Autodesk Inventor part; units mm, degrees
ref_plane "YZ Plane" through (0, 0, 0) normal (1, 0, 0) x (0, 1, 0)
ref_plane "XZ Plane" through (0, 0, 0) normal (0, 1, 0) x (-1, 0, 0)
ref_plane "XY Plane" through (0, 0, 0) normal (0, 0, 1) x (1, 0, 0)
sketch "スケッチ1" plane through (0, 0, 0) normal (0, 0, 1) x (1, 0, 0)
  circle A0 centre (-11.4931, -19.1593) radius 14 construction
  circle A1 centre (16.245, -15.3385) radius 14 construction
  line L0 (-170.915, -81.4118) -> (490.0044, -81.4118)
  line L1 (-197.2268, -33.1593) -> (179.6604, -33.1593) construction
  line L2 (-178.6504, 68.5882) -> (447.0756, 68.5882) construction
  circle A2 centre (-11.4931, -19.1593) radius 14 construction
  circle A3 centre (-21.8854, 6.8407) radius 14 construction
  circle A4 centre (-0.5211, 0.3031) radius 20.05 construction
  circle A5 centre (-0.5211, 0.3031) radius 22.3421 construction
  circle A6 centre (0, 0) radius 22.3421 construction
  circle A7 centre (-0.5211, 0.3031) radius 5.05 construction
  circle A8 centre (19.689, 29.6103) radius 30.55 construction
  circle A9 centre (19.689, 29.6103) radius 10.1 construction
  circle A10 centre (39.672, 58.5882) radius 25.1 construction
  line L3 (-0.5211, 0.3031) -> (39.672, 58.5882) construction
  circle A11 centre (19.689, 29.6103) radius 31.55 construction
  circle A12 centre (19.689, 29.6103) radius 12.1 construction
  circle A13 centre (-0.5211, 0.3031) radius 20.55 construction
  circle A14 centre (-0.5211, 0.3031) radius 6.05 construction
  circle A15 centre (36.8436, 61.4166) radius 4 construction
  circle A16 centre (36.8436, 61.4166) radius 2
  line L4 (36.8436, 61.4166) -> (39.672, 58.5882)
  line L5 (39.672, 58.5882) -> (22.909, 61.4166) construction
  circle A17 centre (22.909, 61.4166) radius 2
  circle A18 centre (22.909, 61.4166) radius 5
  line L6 (28.2635, 50.4737) -> (31.5576, 69.9968) construction
  line L7 (31.5576, 69.9968) -> (51.0806, 66.7027) construction
  line L8 (51.0806, 66.7027) -> (47.7865, 47.1796) construction
  line L9 (47.7865, 47.1796) -> (28.2635, 50.4737) construction
  circle A19 centre (39.672, 58.5882) radius 9
  circle A20 centre (28.2635, 50.4737) radius 2.5
  circle A21 centre (47.7865, 47.1796) radius 2.5
  circle A22 centre (51.0806, 66.7027) radius 2.5
  circle A23 centre (31.5576, 69.9968) radius 2.5
  circle A24 centre (28.2635, 50.4737) radius 5
  line L10 (22.909, 61.4166) -> (36.8436, 61.4166) construction
  line L11 (-26.0808, 51.4166) -> (-426.0808, 51.4166)
  line L12 (-26.0808, 24.4166) -> (23.9192, 24.4166)
  circle A25 centre (39.672, 58.5882) radius 17.5
  circle A26 centre (47.7865, 47.1796) radius 2.1
  circle A27 centre (28.2635, 50.4737) radius 2.1
  circle A28 centre (31.5576, 69.9968) radius 2.1
  circle A29 centre (51.0806, 66.7027) radius 2.1
  circle A30 centre (47.7865, 47.1796) radius 5
  circle A31 centre (31.5576, 69.9968) radius 5
  circle A32 centre (51.0806, 66.7027) radius 5
  circle A33 centre (39.672, 58.5882) radius 19.5
  circle A34 centre (39.672, 58.5882) radius 20.5
  line L13 (20.7504, 89.6882) -> (53.4998, 89.6882)
  line L14 (53.4998, 89.6882) -> (73.6516, 68.9857)
  line L15 (20.7504, 89.6882) -> (-13.977, 39.0272)
  circle A35 centre (-59.2702, 32.0272) radius 5.025 construction
  circle A36 centre (-59.2702, 32.0272) radius 4
  arc A37 (-59.2702, 39.0272) -> (-62.5897, 25.8643) centre (-59.2702, 32.0272) ccw
  line L16 (-59.2702, 39.0272) -> (-13.977, 39.0272)
  line L17 (-62.5897, 25.8643) -> (-36.5547, 11.8407)
  line L18 (-36.5547, 11.8407) -> (-36.5547, -33.1593)
  arc A38 (74.5655, 64.0796) -> (73.6516, 68.9857) centre (70.4271, 65.8469) ccw
  circle A39 centre (8.5193, 63.8863) radius 4.5 construction
  arc A40 (59.4085, 28.8085) -> (59.8353, 29.5856) centre (55.6969, 31.3528) ccw
  circle A41 centre (23.6647, -6.2198) radius 4.5
  circle A42 centre (-16.0241, 34.5272) radius 4.5 construction
  line L19 (59.8353, 29.5856) -> (74.5655, 64.0796)
  line L20 (32.172, 89.6882) -> (32.172, 92.6882)
  line L21 (32.172, 92.6882) -> (47.172, 92.6882)
  line L22 (47.172, 92.6882) -> (47.172, 89.6882)
  line L23 (35.172, 89.6882) -> (35.172, 86.6882)
  line L24 (35.172, 86.6882) -> (44.172, 86.6882)
  line L25 (44.172, 86.6882) -> (44.172, 89.6882)
  circle A43 centre (70.4271, 65.8469) radius 1.5
  circle A44 centre (55.6969, 31.3528) radius 1.5
  circle A45 centre (23.6647, -6.2198) radius 1.5
  circle A46 centre (-16.0241, 34.5272) radius 1.5
  circle A47 centre (8.5193, 63.8863) radius 1.5
  circle A48 centre (-10.0662, 20.4166) radius 4 construction
  circle A49 centre (-10.0662, 20.4166) radius 2
  line L26 (1.9305, -36.1593) -> (16.9305, -36.1593)
  line L27 (16.9305, -36.1593) -> (16.9305, -33.1593)
  line L28 (1.9305, -33.1593) -> (1.9305, -36.1593)
  arc A50 (1.9305, -33.1593) -> (-0.1695, -33.1593) centre (0.8805, -33.1593) ccw
  line L29 (13.9305, -30.1593) -> (13.9305, -33.1593)
  arc A51 (13.9305, -30.1593) -> (11.8305, -30.1593) centre (12.8805, -30.1593) ccw
  line L30 (7.0305, -30.1593) -> (11.8305, -30.1593)
  arc A52 (7.0305, -30.1593) -> (4.9305, -30.1593) centre (5.9805, -30.1593) ccw
  line L31 (4.9305, -33.1593) -> (4.9305, -30.1593)
  arc A53 (4.9305, -33.1593) -> (7.0305, -33.1593) centre (5.9805, -33.1593) ccw
  arc A54 (11.8305, -33.1593) -> (13.9305, -33.1593) centre (12.8805, -33.1593) ccw
  line L32 (-36.5547, -36.1593) -> (-21.5547, -36.1593)
  line L33 (-21.5547, -36.1593) -> (-21.5547, -33.1593)
  arc A55 (-19.4547, -33.1593) -> (-21.5547, -33.1593) centre (-20.5047, -33.1593) ccw
  line L34 (-36.5547, -33.1593) -> (-36.5547, -36.1593)
  arc A56 (-33.5547, -33.1593) -> (-31.4547, -33.1593) centre (-32.5047, -33.1593) ccw
  line L35 (-33.5547, -33.1593) -> (-33.5547, -30.1593)
  arc A57 (-31.4547, -30.1593) -> (-33.5547, -30.1593) centre (-32.5047, -30.1593) ccw
  line L36 (-31.4547, -30.1593) -> (-26.6547, -30.1593)
  arc A58 (-24.5547, -30.1593) -> (-26.6547, -30.1593) centre (-25.6047, -30.1593) ccw
  line L37 (-24.5547, -30.1593) -> (-24.5547, -33.1593)
  arc A59 (-26.6547, -33.1593) -> (-24.5547, -33.1593) centre (-25.6047, -33.1593) ccw
  line L38 (59.4085, 28.8085) -> (16.9305, -33.1593)
  circle A60 centre (-21.8854, 6.8407) radius 5
  circle A61 centre (-11.4931, -19.1593) radius 5
  line L39 (-31.4547, -33.1593) -> (-26.6547, -33.1593)
  line L40 (-19.4547, -33.1593) -> (-0.1695, -33.1593)
  line L41 (7.0305, -33.1593) -> (11.8305, -33.1593)
  line L42 (0.4485, -25.8914) -> (-27.1419, -10.3373) construction
  line L43 (-27.1419, -10.3373) -> (-17.3768, 21.5744) construction
  circle A62 centre (-21.8854, 6.8407) radius 8
  circle A63 centre (-11.4931, -19.1593) radius 8
  circle A64 centre (-19.5445, 14.4905) radius 1.3
  circle A65 centre (-24.2262, -0.8092) radius 1.3
  circle A66 centre (-18.4619, -15.2306) radius 1.3
  circle A67 centre (-4.5242, -23.088) radius 1.3
  circle A68 centre (-0.5211, 0.3031) radius 4.5
  circle A69 centre (19.689, 29.6103) radius 6
  arc A70 (87.3323, 12.0445) -> (87.1264, 18.8999) centre (85.1711, 15.4104) ccw
  line L44 (16.9305, -33.1593) -> (87.3323, 12.0445)
  line L45 (87.1264, 18.8999) -> (61.4227, 33.3027)
  circle A71 centre (85.1711, 15.4104) radius 2
  dimension "d0" = 150
  dimension "d1" = 28
  dimension "d2" = 28
  dimension "d3" = 40.1
  dimension "d4" = 10.1
  dimension "d5" = 61.1
  dimension "d6" = 20.2
  dimension "d7" = 50.2
  dimension "d8" = 10
  dimension "d9" = 2
  dimension "d10" = 1
  dimension "d11" = 2
  dimension "d12" = 0.5
  dimension "d13" = 1
  dimension "d14" = 40
  dimension "d15" = 8
  dimension "d16" = 4
  dimension "d17" = 4
  dimension "d18" = 45
  dimension "d19" = 17
  dimension "d20" = 4
  dimension "d21" = 3
  dimension "d22" = 1
  dimension "d23" = 5
  dimension "d24" = 5
  dimension "d25" = 5
  dimension "d26" = 5
  dimension "d27" = 10
  dimension "d28" = 400
  dimension "d29" = 10
  dimension "d30" = 50
  dimension "d31" = 50
  dimension "d32" = 27
  dimension "d33" = 27
  dimension "d34" = 35
  dimension "d35" = 4.2
  dimension "d36" = 4.2
  dimension "d37" = 4.2
  dimension "d38" = 4.2
  dimension "d39" = 10
  dimension "d40" = 10
  dimension "d41" = 10
  dimension "d42" = 2
  dimension "d43" = 1
  dimension "d44" = 8
  dimension "d45" = 3
  dimension "d46" = 4
  dimension "d47" = 9
  dimension "d48" = 9
  dimension "d49" = 9
  dimension "d50" = 9
  dimension "d51" = 9
  dimension "d52" = 3
  dimension "d53" = 15
  dimension "d54" = 3
  dimension "d55" = 9
  dimension "d56" = 3
  dimension "d57" = 7.5
  dimension "d58" = 3
  dimension "d59" = 3
  dimension "d60" = 3
  dimension "d61" = 3
  dimension "d62" = 3
  dimension "d63" = 8
extrude "押し出し1" add sketch "スケッチ1" along normal blind 4 contours A17 A25 | A17 A25 A18 | A25 A31 A19 A24 A18 | A25 A31 | A24 A25 | A25 A32 A19 A31 | A19 A30 A25 A24 | A25 A32 | A32 A25 A30 A19 | A30 A25 | A20 | A21 | A22 | A23 picked at (23.2356, 61.3111) picked at (31.8427, 73.6117) picked at (27.4228, 46.9526) picked at (51.9213, 70.2238) picked at (47.5014, 43.5647)
properties part number "横回転首振り最終段カム" material "アルミニウム 7075"
Geometry check sheet. Reference: the model listing, model coordinates, mm. Coordinates: 2 decimals unless noted, no trailing zeros. Order: outer loops, then holes, each group sorted by start corner. A loop starts at its lowest first (then second) coordinate and runs counter-clockwise, first axis right, second up.
Item 1: Section check D-D (y = 44.5). Enter the section's corners in (x, z).
Item 2: Section check C-C (z = 2). Enter the section's corners in (x, y), plus the area to 3 significant figures.
Item 3: Scan lines: line 1 along X through (y, z) = (58.5, 3.1); line 2 along Y through (x, z) = (33, 1.35); line 3 along Y through (x, z) = (49.5, 3.45). Record each from-to range of solid material in increasing order.
Item 4: Depth check by flat-ended pin: pin 1 (2.5 mm diameter, centred on x = 51.08, y = 66.7, fed in from -Z); pin 2 (2 mm diameter, centred on y = 50.5, z = 3, fed in from -X). Enter the tip coordinate at first touch or a pass-through.
Item 5: Section check A-A (y = 60). Enter the section's corners in (x, z).
Item 6: Section check B-B (x = 42). Enter the section's corners in (y, z).
Item 7: Mould release check, pull along Y, two halves, no side actions. Record for faces 1 (the flat face through (36, 67, 4)), 2 (the cylindrical face through (26.774, 46.761, 1.972)), 3 (the cylindrical face through (26.597, 51.752, 1.972)): released by +Y, released by -Y, zero draft, split by the parting line, or undercut.
Check sheet entries:
1. outline: (29.29, 0) - (50.05, 0) - (50.05, 4) - (29.29, 4) - close
2. outline: circle Ø35 at (39.67, 58.59); hole circle Ø4.2 at (28.26, 50.47); hole circle Ø4.2 at (31.56, 70); hole circle Ø18 at (39.67, 58.59); hole circle Ø4.2 at (47.79, 47.18); hole circle Ø4.2 at (51.08, 66.7)
2. area: 652 mm2
3. line 1: x = 22.17 to 30.67, 48.67 to 57.17
3. line 2: y = 42.41 to 52.55, 64.63 to 68.47, 71.52 to 74.77
3. line 3: y = 44.11 to 45.97, 48.39 to 65.32, 68.09 to 73.07
4. pin 1: passes through
4. pin 2: stops at x = 23.67
5. outline: (22.23, 0) - (30.78, 0) - (30.78, 4) - (22.23, 4) - close; (48.56, 0) - (57.11, 0) - (57.11, 4) - (48.56, 4) - close
6. outline: (41.24, 0) - (49.89, 0) - (49.89, 4) - (41.24, 4) - close; (67.28, 0) - (75.93, 0) - (75.93, 4) - (67.28, 4) - close
7. face 1: zero draft
7. face 2: split by the parting line
7. face 3: undercut
